The model under review builds one solid part; all positions refer to its coordinate system, in mm. Coordinates: 2 decimals unless noted, no trailing zeros. Write item = value, one per line. Start each with the question number.
Q1. Wall thickness on probe 1 along Y at (x, z) = (0, 0); probe 2 along X at (y, z) = (3.5, -0.05); probe 3 along Y at (x, z) = (1.25, -0.05): over which ranges is each line inside the solid? List them lowest first.
Q2. Clearance check with a flat-ended pin moving along its axis: pin 1 Ø5 at (x, y) = (1, -4) entering from +Z. State where the tip first meets the part, or that it passes through.
Q3. Mouldability with a two-part tool opening along X and no side actions: class faces 1 (the face through (-5, 4, -0.229)), 2 (the face through (5.55, -3.09, 0)) as released by +X, released by -X, zero draft, split by the parting line, or undercut.
from build123d import *

# Parameters (mm, degrees)
EXTRUDE1_DEPTH = 0.2286
FILLET1_R      = 0.20574


with BuildPart() as part:
    # Sketch2 → Extrude1 (new, symmetric)
    with BuildSketch(Plane.XY):
        with BuildLine():
            Line((6.280836093, -1.682944959), (6.832862703, -1.830860043))
            ThreePointArc((6.832862703, -1.830860043), (-7.0739, 0), (6.832862703, 1.830860043))
            Line((6.832862703, 1.830860043), (5.728809483, 1.535029875))
            ThreePointArc((5.728809483, 1.535029875), (-5.754578473, 1.435409842), (4.336748761, -4.045761362))
            ThreePointArc((4.336748761, -4.045761362), (5.564729157, -3.074933786), (6.280836093, -1.682944959))
        make_face()
    extrude(amount=EXTRUDE1_DEPTH, both=True)

    # Fillet1
    fillet1_edges = [part.edges().sort_by_distance(p)[0] for p in [
        (-7.0739, 0, 0.2286),
        (-5.754578473, 1.435409842, 0.2286),
        (-7.0739, 0, -0.2286),
        (-5.754578473, 1.435409842, -0.2286),
    ]]
    fillet(fillet1_edges, radius=FILLET1_R)


solid = part.part
Returned:
q1.probe_1 = -7.07 to -5.93, 5.93 to 7.07
q1.probe_2 = -6.15 to -4.79, 4.79 to 6.15
q1.probe_3 = -6.96 to -5.8, 5.8 to 6.96
q2.pin_1 = 0.23
q3.face_1 = zero draft
q3.face_2 = undercut
